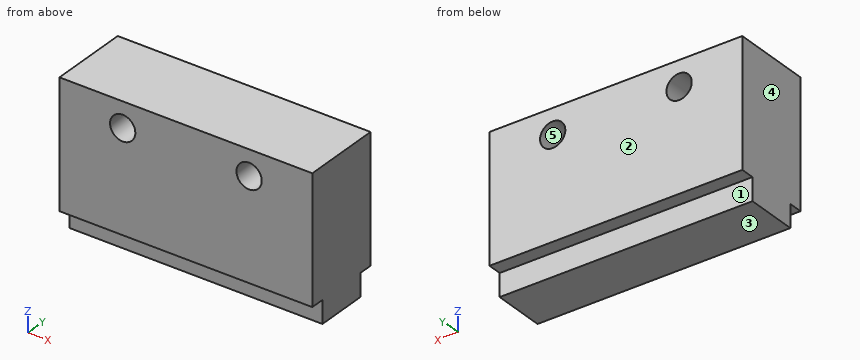
from build123d import *

# Parameters (mm, degrees)
SKETCH1_W           = 20
SKETCH1_H           = 10
BOSS_EXTRUDE1_DEPTH = 6.3
SKETCH2_W           = 20
SKETCH2_H           = 4.1
BOSS_EXTRUDE2_DEPTH = 1.8
SKETCH3_R           = 1
CUT_EXTRUDE1_DEPTH  = 25.060964237


with BuildPart() as part:
    # Sketch1 → Boss-Extrude1 (new body)
    with BuildSketch(Plane(origin=(0, 0, 0), x_dir=(1, 0, 0), z_dir=(0, 1, 0))):
        with Locations((10, 5)):
            Rectangle(SKETCH1_W, SKETCH1_H)
    extrude(amount=BOSS_EXTRUDE1_DEPTH)

    # Sketch2 → Boss-Extrude2 (add)
    with BuildSketch(Plane(origin=(0, 0, -10), x_dir=(-1, 0, 0), z_dir=(0, 0, -1))):
        with Locations((-10, 3.15)):
            Rectangle(SKETCH2_W, SKETCH2_H)
    extrude(amount=BOSS_EXTRUDE2_DEPTH)

    # Sketch3 → Cut-Extrude1 (cut, through all)
    with BuildSketch(Plane(origin=(0, 6.3, 0), x_dir=(1, 0, 0), z_dir=(0, 1, 0))):
        with Locations(Location((5, 2, 0), (0, 0, 270))):
            Circle(SKETCH3_R)
        with Locations(Location((15, 2, 0), (0, 0, 270))):
            Circle(SKETCH3_R)
    extrude(amount=-CUT_EXTRUDE1_DEPTH, mode=Mode.SUBTRACT)


solid = part.part
Design review of the part built by this model. Coordinates are the model's own, in mm. Face numbers are marked on the shaded views. A direction names the side the tool comes from. Round coordinates to 2 decimals unless told otherwise and drop trailing zeros. Write each loop counter-clockwise with the first axis right and the second up, starting at its lowest first coordinate (ties: lowest second). Pieces come first, ordered by that corner, then holes. Notation, with made-up numbers: (-24, -30) - (-6, -30) arc R23 cw to (-6, -22) - close; hole circle Ø7 at (49.25, 10.25). An arc over 180 degrees is marked (long way). Use a Markdown table: item, result. Add a question column.
1. We need section D-D (x = 2). State the section outline as (y, z) points, then the cut area to 3 significant figures.
2. Wall thickness on probe 1 along X at (y, z) = (1.5, -2); probe 2 along X at (y, z) = (3.75, -2.5); probe 3 along Y at (x, z) = (18, -10.75): over which ranges is each line inside the solid? List them lowest first.
3. We need section C-C (y = 5.5). State the section outline as (x, z) points.
4. For the marked faces 1 and 2, list the 3-axis set-ups (+Z, -Z, +X, -X, +Y, -Y) from which the entire face can be reached by the end or side of a thin tool; tool diameter is ignored.
5. Mouldability with a two-part tool opening along Z and no side actions: class the marked faces 3, 4 and 5 as +Z half, -Z half, draft (parallel to the pull), parting line (faces both ways), or undercut.
6. We need section A-A (z = -2). State the section outline as (x, y) points, then the cut area to 3 significant figures.
7. Clearance check with a flat-ended pin moving along its axis: pin 1 (1.4 mm diameter, centred on x = 13.5, z = -11, fed in from -Y). State where the tip first meets the part, or that it passes through.
8. We need section B-B (x = 5). State the section outline as (y, z) points.
Output:
| question | item | result |
|---|---|---|
| 1 | outline | (0, -10) - (1.1, -10) - (1.1, -11.8) - (5.2, -11.8) - (5.2, -10) - (6.3, -10) - (6.3, 0) - (0, 0) - close |
| 1 | area | 70.4 mm2 |
| 2 | probe 1 | x = 0 to 4, 6 to 14, 16 to 20 |
| 2 | probe 2 | x = 0 to 4.13, 5.87 to 14.13, 15.87 to 20 |
| 2 | probe 3 | y = 1.1 to 5.2 |
| 3 | outline | (0, -10) - (20, -10) - (20, 0) - (0, 0) - close; hole circle Ø2 at (5, -2); hole circle Ø2 at (15, -2) |
| 4 | face 1 | -Z, +X, -X, +Y |
| 4 | face 2 | +Z, -Z, +X, -X, +Y |
| 5 | face 3 | -Z half |
| 5 | face 4 | draft |
| 5 | face 5 | undercut |
| 6 | outline | (0, 0) - (4, 0) - (4, 6.3) - (0, 6.3) - close; (6, 0) - (14, 0) - (14, 6.3) - (6, 6.3) - close; (16, 0) - (20, 0) - (20, 6.3) - (16, 6.3) - close |
| 6 | area | 101 mm2 |
| 7 | pin 1 | stops at y = 1.1 |
| 8 | outline | (0, -10) - (1.1, -10) - (1.1, -11.8) - (5.2, -11.8) - (5.2, -10) - (6.3, -10) - (6.3, -3) - (0, -3) - close; (0, -1) - (6.3, -1) - (6.3, 0) - (0, 0) - close |
